The model under review builds one solid part; all positions refer to its coordinate system, in mm. Face numbers are marked on the shaded views. Coordinates: 2 decimals unless noted, no trailing zeros. Write each loop counter-clockwise with the first axis right and the second up, starting at its lowest first coordinate (ties: lowest second). Pieces come first, ordered by that corner, then holes. Notation, with made-up numbers: (47, 84.5) - (100, 84.5) arc R32 ccw to (100, 111.5) - close; hole circle Ø11 at (36, -8.5). An arc over 180 degrees is marked (long way). Return JSON: item names as keys, results as strings. Group by question number.
(1) Draft analysis for pull direction X (two halves, no side actions). For the marked faces 1 and 2, state which applies: released by +X, released by -X, zero draft, split by the parting line, or undercut.
(2) We need section C-C on x = 27. State the section outline as (y, z) points.
(3) For pin 1 Ø1 at (x, z) = (2, 91) entering from +Y; pin 2 Ø12 at (x, z) = (17.5, 148) entering from -Y; pin 3 Ø0.6 at (y, z) = (2.5, 51.5) entering from +X; pin 4 Ø1 at (y, z) = (0.5, 137.5) entering from -X, all flat-tipped, find the tip position at first contact; note any pin that passes through.
(4) We need section B-B on z = 16.5. State the section outline as (x, y) points, then the cut area to 3 significant figures.
(5) To check wall thickness, follow L1, parallel to X at y = 2.75, z = 165; L2, parallel to Y at x = 26, z = 161.5; L3, parallel to X at y = 0.5, z = 23. State the ranges of each line that lie inside material, in increasing order. Write a range as from..to.
(6) We need section A-A on y = 2.7. State the section outline as (x, z) points.
```python
from build123d import *

# Parameters (mm, degrees)
PAD_DEPTH   = 200
FILLET_R    = 1.5
FILLET001_R = 1.5
FILLET002_R = 0.5
FILLET003_R = 0.5
FILLET004_R = 0.5
FILLET005_R = 0.5


with BuildPart() as part:
    # Sketch → Pad (new body)
    with BuildSketch(Plane.XY):
        Polygon((0, 0), (5, 0), (5, 4), (30, 4), (30, 0), (35, 0), (35, 1), (31, 1), (31, 5), (4, 5), (4, 1), (0, 1), align=None)
    extrude(amount=PAD_DEPTH)

    # Fillet
    fillet_edges = [part.edges().sort_by_distance(p)[0] for p in [
        (4, 5, 100),
    ]]
    fillet(fillet_edges, radius=FILLET_R)

    # Fillet001
    fillet001_edges = [part.edges().sort_by_distance(p)[0] for p in [
        (31, 5, 100),
        (30, 0, 100),
        (5, 0, 100),
    ]]
    fillet(fillet001_edges, radius=FILLET001_R)

    # Fillet002
    fillet002_edges = [part.edges().sort_by_distance(p)[0] for p in [
        (5, 4, 100),
    ]]
    fillet(fillet002_edges, radius=FILLET002_R)

    # Fillet003
    fillet003_edges = [part.edges().sort_by_distance(p)[0] for p in [
        (31, 1, 100),
    ]]
    fillet(fillet003_edges, radius=FILLET003_R)

    # Fillet004
    fillet004_edges = [part.edges().sort_by_distance(p)[0] for p in [
        (4, 1, 100),
    ]]
    fillet(fillet004_edges, radius=FILLET004_R)

    # Fillet005
    fillet005_edges = [part.edges().sort_by_distance(p)[0] for p in [
        (30, 4, 100),
    ]]
    fillet(fillet005_edges, radius=FILLET005_R)


solid = part.part
```
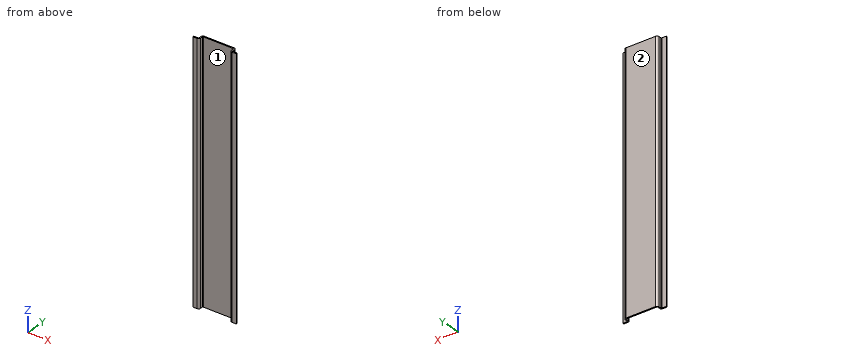
Ans:
{
 "1": {"face 1": "undercut", "face 2": "zero draft"},
 "2": {"outline": "(4, 0) - (5, 0) - (5, 200) - (4, 200) - close"},
 "3": {"pin 1": "y = 1", "pin 2": "y = 4", "pin 3": "x = 31", "pin 4": "x = 0"},
 "4": {"outline": "(0, 0) - (3.5, 0) arc R1.5 ccw to (5, 1.5) - (5, 3.5) arc R0.5 cw to (5.5, 4) - (29.5, 4) arc R0.5 cw to (30, 3.5) - (30, 1.5) arc R1.5 ccw to (31.5, 0) - (35, 0) - (35, 1) - (31.5, 1) arc R0.5 cw to (31, 1.5) - (31, 3.5) arc R1.5 ccw to (29.5, 5) - (5.5, 5) arc R1.5 ccw to (4, 3.5) - (4, 1.5) arc R0.5 cw to (3.5, 1) - (0, 1) - close", "area": "41.3 mm²"},
 "5": {"L1": "4..5, 30..31", "L2": "4..5", "L3": "0..4.62, 30.38..35"},
 "6": {"outline": "(4, 0) - (5, 0) - (5, 200) - (4, 200) - close; (30, 0) - (31, 0) - (31, 200) - (30, 200) - close"}
}
